Verification items for the finished model (mm, model axes). A direction names the side the tool comes from. Give positions to 0.01 mm unless a question says otherwise; leave off trailing zeros. Loops run counter-clockwise (first coordinate to the right, second up) from the corner with the lowest first, then second, coordinate; pieces in that order, holes last. Notation, with made-up numbers: M 75,68 L 130,68 A21 cw 130,85 Z; hole C 7,2.5 d6. An arc over 180 degrees is marked long. Use CSV: the item, a comma, the result in double quotes.
from build123d import *
from OCP.BRepFilletAPI import BRepFilletAPI_MakeChamfer

# Parameters (mm, degrees)
BOSS_EXTRUDE1_DEPTH = 27.432
CHAMFER1_SIZE       = 0.254
CHAMFER1_SIZE2      = 0.146646968


# Read off the part's stored shape, not the designer's step: Cut-Revolve4
with BuildPart() as part:
    # Sketch3 → Boss-Extrude1 (new body)
    with BuildSketch(Plane(origin=(0, 0, 0), x_dir=(1, 0, 0), z_dir=(0, 1, 0))):
        Polygon((4.7625, 2.749630657), (0, 5.499261314), (-4.7625, 2.749630657), (-4.7625, -2.749630657), (0, -5.499261314), (4.7625, -2.749630657), align=None)
    extrude(amount=BOSS_EXTRUDE1_DEPTH)

    # Cut-Revolve4 outline → Cut-Revolve4 (revolve, cut)
    with BuildSketch(Plane.XY):
        Polygon((4.6609, 9.18188181), (3.1369, 8.302), (5.499261314, 8.302), (5.499261314, 27.432), (2.54, 27.432), (2.54, 16.302), (3.1369, 16.302), (4.6609, 15.42211819), align=None)
        Polygon((0.99695, 21.082), (2, 21.082), (2, 27.432), (0, 27.432), (0, 1.391072642), (0.99695, 1.92116036), align=None)
    revolve(axis=Axis((0, 0, 0), (0, 1, 0)), mode=Mode.SUBTRACT)

    # Chamfer1: one chamfer whose edges measure the first distance from different faces: ONE call of the kernel's chamfer builder (chamfer() names one face for all edges)
    chamfer1_edges_1 = [part.edges().sort_by_distance(p)[0] for p in [
        (-2.54, 27.432, 0),
    ]]
    chamfer1_side_1 = [part.faces().sort_by_distance(p)[0] for p in [
        (-2.468157951, 27.432, 0),
    ]]
    chamfer1_edges_2 = [part.edges().sort_by_distance(p)[0] for p in [
        (-2, 27.432, 0),
    ]]
    chamfer1_side_2 = [part.faces().sort_by_distance(p)[0] for p in [
        (-2, 24.257, 0),
    ]]
    chamfer1 = BRepFilletAPI_MakeChamfer(part.part.solid().wrapped)
    for e in chamfer1_edges_1:
        chamfer1.Add(CHAMFER1_SIZE, CHAMFER1_SIZE2, e.wrapped, chamfer1_side_1[0].wrapped)  # the first distance lies on this face
    for e in chamfer1_edges_2:
        chamfer1.Add(CHAMFER1_SIZE, CHAMFER1_SIZE2, e.wrapped, chamfer1_side_2[0].wrapped)  # the first distance lies on this face
    add(Compound.cast(chamfer1.Shape()), mode=Mode.REPLACE)

    # Sketch4 → Cut-Revolve5 (revolve, cut)
    with BuildSketch(Plane.XY, mode=Mode.PRIVATE) as cut_revolve5_sk:
        Polygon((-0.35, 0.762), (-0.5, 0.762), (-3, 2.091273579), (-3, 5.762), (-6.107414125, 5.762), (-6.107414125, 0), (0, 0), (0, 1.524), (-0.35, 1.524), align=None)
    revolve(cut_revolve5_sk.sketch.rotate(Axis((0, 0, 0), (0, 1, 0)), 270), axis=Axis((0, 0, 0), (0, 1, 0)), mode=Mode.SUBTRACT)


solid = part.part
(1) Depth check by flat-ended pin: pin 1 Ø1.5 at (x, z) = (-3.5, 3) entering from -Y; pin 2 Ø3 at (x, z) = (2, 4.5) entering from +Y; pin 3 Ø1.5 at (x, y) = (-1, 13.5) entering from +Z. Enter the tip coordinate at first touch or a pass-through.
Calculated:
pin 1,"stops at y = 5.76"
pin 2,"stops at y = 16.14"
pin 3,"stops at z = 4.65"
(2) Mould release check, pull along X, two halves, no side actions. Record for faces 6 (the flat face through (2.41, 7.01, -4.11)), 7 (the flat face through (-1, 21.082, 1)), 8 (the cylindrical face through (-0.33, 21.72, -2.52)): released by +X, released by -X, zero draft, split by the parting line, or undercut.
Calculated:
face 6,"released by +X"
face 7,"undercut"
face 8,"split by the parting line"
(3) Scan lines: L1, parallel to Z at x = 0, y = 16.5; L2, parallel to X at y = 10.5, z = 0; L3, parallel to X at y = 25.75, z = 0. Record each from-to range of solid material in increasing order. Write a range as from..to.
Calculated:
L1,"z = -2.54..-1, 1..2.54"
L2,"x = -4.66..-1, 1..4.66"
L3,"x = -2.54..-2, 2..2.54"
(4) Section check A-A on y = 17.5. Record the cut outline in (x, z).
Calculated:
outline,"C 0,0 d5.08; hole C 0,0 d1.99"
(5) Tool access check on faces 1 (the cylindrical face through (0.95, 11.64, -0.3)), 2 (the cylindrical face through (-0.9, 3.95, -2.86)), 3 (the flat face through (3.24, 8.302, 1.15)), 4 (the flat face through (-4.762, 7, 0)), 5 (the flat face through (4.762, 7, 0)). Record the directions out of +Z, -Z, +X, -X, +Y, -Y that give a thin tool (end or side, any length) a straight path to the whole face; none if there is none.
Calculated:
face 1,"+Y"
face 2,"-Y"
face 3,"none"
face 4,"+Z, -Z, -X, +Y, -Y"
face 5,"+Z, -Z, +X, +Y, -Y"
(6) Section check B-B on y = 3.25. Record the cut outline in (x, z).
Calculated:
outline,"C 0,0 d6; hole C 0,0 d1.99"
